```python
from build123d import *

# Parameters (mm, degrees)
ESQUISSE1_W                  = 34
ESQUISSE1_H                  = 80
BOSS_EXTRU_1_DEPTH           = 8
ESQUISSE2_R                  = 1.25
ENL_V_MAT_EXTRU_1_DEPTH      = 1
ENL_V_MAT_EXTRU_1_DEPTH_BACK = 9
ESQUISSE3_R                  = 2.25
ENL_V_MAT_EXTRU_2_DEPTH      = 1
ENL_V_MAT_EXTRU_2_DEPTH_BACK = 9
ESQUISSE4_R                  = 4
ENL_V_MAT_EXTRU_3_DEPTH      = 4
CONG_1_R                     = 5


with BuildPart() as part:
    # Esquisse1 → Boss.-Extru.1 (new body)
    with BuildSketch(Plane.XY):
        with Locations((17, 40)):
            Rectangle(ESQUISSE1_W, ESQUISSE1_H)
    extrude(amount=BOSS_EXTRU_1_DEPTH)

    # Esquisse2 → Enlèv. mat.-Extru.1 (cut, two sides)
    with BuildSketch(Plane.XY.offset(8)) as enl_v_mat_extru_1_sk:
        with Locations((17, 17.5)):
            Circle(ESQUISSE2_R)
        with Locations((17, 42.5)):
            Circle(ESQUISSE2_R)
        with Locations((17, 67.5)):
            Circle(ESQUISSE2_R)
        with Locations((17, 92.5)):
            Circle(ESQUISSE2_R)
        with Locations((17, 117.5)):
            Circle(ESQUISSE2_R)
        with Locations((17, 142.5)):
            Circle(ESQUISSE2_R)
        with Locations((17, 167.5)):
            Circle(ESQUISSE2_R)
        with Locations((17, 192.5)):
            Circle(ESQUISSE2_R)
    extrude(amount=ENL_V_MAT_EXTRU_1_DEPTH, mode=Mode.SUBTRACT)
    extrude(enl_v_mat_extru_1_sk.sketch, amount=-ENL_V_MAT_EXTRU_1_DEPTH_BACK, mode=Mode.SUBTRACT)

    # Esquisse3 → Enlèv. mat.-Extru.2 (cut, two sides)
    with BuildSketch(Plane.XY.offset(8)) as enl_v_mat_extru_2_sk:
        with Locations((6, 16)):
            Circle(ESQUISSE3_R)
        with Locations((28, 16)):
            Circle(ESQUISSE3_R)
        with Locations((28, 72)):
            Circle(ESQUISSE3_R)
        with Locations((6, 72)):
            Circle(ESQUISSE3_R)
    extrude(amount=ENL_V_MAT_EXTRU_2_DEPTH, mode=Mode.SUBTRACT)
    extrude(enl_v_mat_extru_2_sk.sketch, amount=-ENL_V_MAT_EXTRU_2_DEPTH_BACK, mode=Mode.SUBTRACT)

    # Esquisse4 → Enlèv. mat.-Extru.3 (cut)
    with BuildSketch(Plane.XY.offset(8)):
        with Locations((6, 16)):
            Circle(ESQUISSE4_R)
        with Locations((28, 16)):
            Circle(ESQUISSE4_R)
        with Locations((6, 72)):
            Circle(ESQUISSE4_R)
        with Locations((28, 72)):
            Circle(ESQUISSE4_R)
    extrude(amount=-ENL_V_MAT_EXTRU_3_DEPTH, mode=Mode.SUBTRACT)

    # Congé1
    cong_1_edges = [part.edges().sort_by_distance(p)[0] for p in [
        (0, 80, 4),
        (34, 80, 4),
        (34, 0, 4),
        (0, 0, 4),
    ]]
    fillet(cong_1_edges, radius=CONG_1_R)


solid = part.part
```
Geometry check sheet. Reference: the model listing, model coordinates, mm. A direction names the side the tool comes from. Coordinates: 2 decimals unless noted, no trailing zeros. Order: outer loops, then holes, each group sorted by start corner. A loop starts at its lowest first (then second) coordinate and runs counter-clockwise, first axis right, second up.
Q1. Tool access check on faces 1 (the face through (8, 14, 4)), 2 (the face through (27.512, 69.804, 2.028)). Record the directions out of +Z, -Z, +X, -X, +Y, -Y that give a thin tool (end or side, any length) a straight path to the whole face; none if there is none.
Reply:
face 1: +Z
face 2: +Z, -Z
Q2. Thickness scan on probe 1 along Y at (x, z) = (17, 5.25); probe 2 along Y at (x, z) = (28, 5); probe 3 along Y at (x, z) = (28, 2.3). Record the ranges inside material, lowest first.
Reply:
probe 1: y = 0 to 16.25, 18.75 to 41.25, 43.75 to 66.25, 68.75 to 80
probe 2: y = 0 to 12, 20 to 68, 76 to 80
probe 3: y = 0 to 13.75, 18.25 to 69.75, 74.25 to 80
Q3. Sectioned sample at B-B on y = 72. Record the cut outline in (x, z).
Reply:
outline: (0, 0) - (3.75, 0) - (3.75, 4) - (2, 4) - (2, 8) - (0, 8) - close; (8.25, 0) - (25.75, 0) - (25.75, 4) - (24, 4) - (24, 8) - (10, 8) - (10, 4) - (8.25, 4) - close; (30.25, 0) - (34, 0) - (34, 8) - (32, 8) - (32, 4) - (30.25, 4) - close
Q4. Depth check by flat-ended pin: pin 1 Ø7 at (x, y) = (28, 16) entering from +Z; pin 2 Ø1.5 at (x, z) = (30.5, 6) entering from +Y. Enter the tip coordinate at first touch or a pass-through.
Reply:
pin 1: stops at z = 4
pin 2: stops at y = 79.94
Q5. Draft check along Y on faces 3 (the face through (17, 41, 8)), 4 (the face through (25.05, 18.7, 6.03)), 5 (the face through (32, 79, 4)). Enter one of: released by +Y, released by -Y, zero draft, split by the parting line, or undercut.
Reply:
face 3: zero draft
face 4: undercut
face 5: released by +Y
Q6. Sectioned sample at A-A on x = 17. Record the cut outline in (y, z).
Reply:
outline: (0, 0) - (16.25, 0) - (16.25, 8) - (0, 8) - close; (18.75, 0) - (41.25, 0) - (41.25, 8) - (18.75, 8) - close; (43.75, 0) - (66.25, 0) - (66.25, 8) - (43.75, 8) - close; (68.75, 0) - (80, 0) - (80, 8) - (68.75, 8) - close
Q7. Sectioned sample at C-C on y = 17.5. Record the cut outline in (x, z).
Reply:
outline: (0, 0) - (4.32, 0) - (4.32, 4) - (2.29, 4) - (2.29, 8) - (0, 8) - close; (7.68, 0) - (15.75, 0) - (15.75, 8) - (9.71, 8) - (9.71, 4) - (7.68, 4) - close; (18.25, 0) - (26.32, 0) - (26.32, 4) - (24.29, 4) - (24.29, 8) - (18.25, 8) - close; (29.68, 0) - (34, 0) - (34, 8) - (31.71, 8) - (31.71, 4) - (29.68, 4) - close
